Verification items for the finished model (mm, model axes). Coordinates: 2 decimals unless noted, no trailing zeros. Write each loop counter-clockwise with the first axis right and the second up, starting at its lowest first coordinate (ties: lowest second). Pieces come first, ordered by that corner, then holes. Notation, with made-up numbers: M 29.5,-8 L 50.5,-8 A17 ccw 50.5,1 Z; hole C 15,-12 d6. An arc over 180 degrees is marked long. One line per item, written item: value.
```python
from build123d import *

# Parameters (mm, degrees)
F0_R          = 18.5
F0_R_2        = 12.5
F1_DEPTH      = 5
F1_DEPTH_BACK = 5
F2_SIZE       = 0.5


with BuildPart() as f1:
    # F0 (on Top) → F1 (new body, two sides)
    with BuildSketch(Plane.XY) as f1_sk:
        Circle(F0_R)
        Circle(F0_R_2, mode=Mode.SUBTRACT)
    extrude(amount=F1_DEPTH)
    extrude(f1_sk.sketch, amount=-F1_DEPTH_BACK)

    # F2
    f2_edges = [f1.edges().sort_by_distance(p)[0] for p in [
        (-12.5, 0, -5),
        (-18.5, 0, -5),
        (-12.5, 0, 5),
        (-18.5, 0, 5),
    ]]
    chamfer(f2_edges, length=F2_SIZE)


solid = f1.part
```
Item 1: Go/stop test with flat-tipped pins: P1, Ø4, axis at y = 14.5, z = -0.5, coming from the -X side; P2, Ø6, axis at y = 4, z = -2.5, coming from the -X side; P3, Ø4, axis at y = 7.5, z = -2, coming from the +X side. Record where each tip stops, or that it passes through.
The answers:
P1: stops at x = -13.64
P2: stops at x = -18.47
P3: stops at x = 17.66
Item 2: Cross-section at A-A, the plane x = 0. Enter the section's corners in (y, z).
The answers:
outline: M -18.5,-4.5 L -18,-5 L -13,-5 L -12.5,-4.5 L -12.5,4.5 L -13,5 L -18,5 L -18.5,4.5 Z; M 12.5,-4.5 L 13,-5 L 18,-5 L 18.5,-4.5 L 18.5,4.5 L 18,5 L 13,5 L 12.5,4.5 Z
Item 3: Scan lines: line 1 (Y direction, x = 0, z = -1.45); line 2 (Y direction, x = -5.5, z = 4); line 3 (X direction, y = 0.5, z = -3.25). Record each from-to range of solid material in increasing order.
The answers:
line 1: y = -18.5 to -12.5, 12.5 to 18.5
line 2: y = -17.66 to -11.22, 11.22 to 17.66
line 3: x = -18.49 to -12.49, 12.49 to 18.49
Item 4: Cross-section at C-C, the plane z = -3.5. Enter the section's corners in (x, y), and give its area (3 significant figures).
The answers:
outline: C 0,0 d37; hole C 0,0 d25
area: 584 mm²
